from build123d import *

# Parameters (mm, degrees)
SKETCH1_R           = 4
SKETCH1_R_2         = 1.85
BOSS_EXTRUDE1_DEPTH = 2.3368


with BuildPart() as part:
    # Sketch1 → Boss-Extrude1 (new body)
    with BuildSketch(Plane.XY):
        with BuildLine():
            Line((-29.579916475, -5.002853321), (-33.915090683, 20.629337502))
            ThreePointArc((-33.915090683, 20.629337502), (-33.978735385, 21.133158673), (-34, 21.640538448))
            Line((-34, 21.640538448), (-34, 55.247304326))
            ThreePointArc((-34, 55.247304326), (-33.538424872, 57.567799195), (-32.223970118, 59.535019756))
            Line((-32.223970118, 59.535019756), (-9.899494937, 81.859494937))
            ThreePointArc((-9.899494937, 81.859494937), (0, 85.96), (9.899494937, 81.859494937))
            Line((9.899494937, 81.859494937), (32.223970118, 59.535019756))
            ThreePointArc((32.223970118, 59.535019756), (33.538424872, 57.567799195), (34, 55.247304326))
            Line((34, 55.247304326), (34, 21.640538448))
            ThreePointArc((34, 21.640538448), (33.978735385, 21.133158673), (33.915090683, 20.629337502))
            Line((33.915090683, 20.629337502), (29.579916475, -5.002853321))
            ThreePointArc((29.579916475, -5.002853321), (0, -30), (-29.579916475, -5.002853321))
        make_face()
        Circle(SKETCH1_R, mode=Mode.SUBTRACT)
        with Locations((0, 8)):
            Circle(SKETCH1_R_2, mode=Mode.SUBTRACT)
        with Locations((-8, 0)):
            Circle(SKETCH1_R_2, mode=Mode.SUBTRACT)
        with Locations((0, -8)):
            Circle(SKETCH1_R_2, mode=Mode.SUBTRACT)
        with Locations((8, 0)):
            Circle(SKETCH1_R_2, mode=Mode.SUBTRACT)
        with Locations((0, 71.96)):
            Circle(SKETCH1_R, mode=Mode.SUBTRACT)
        with Locations((-29.2625, 32)):
            Circle(SKETCH1_R_2, mode=Mode.SUBTRACT)
        with Locations((29.2625, 43.5)):
            Circle(SKETCH1_R_2, mode=Mode.SUBTRACT)
        with Locations((29.2625, 32)):
            Circle(SKETCH1_R_2, mode=Mode.SUBTRACT)
        with Locations((-29.2625, 43.5)):
            Circle(SKETCH1_R_2, mode=Mode.SUBTRACT)
    extrude(amount=BOSS_EXTRUDE1_DEPTH)


solid = part.part
Geometry: final body of the model. Coordinates: model frame, mm. Coordinates: 2 decimals unless noted, no trailing zeros. Loops run counter-clockwise (first coordinate to the right, second up) from the corner with the lowest first, then second, coordinate; pieces in that order, holes last. Notation, with made-up numbers: M -8,50 L 44,50 A29 cw 44,73 Z; hole C -17.75,65.25 d8. An arc over 180 degrees is marked long. One line per item, written item: value. Start each with the question number.
1) Pin query (flat end, axial travel): P1, Ø2, axis at x = 0, y = 8, coming from the -Z side; P2, Ø4.5, axis at x = 29.26, y = 43.5, coming from the +Z side. Return the tip coordinate at first contact, or that it passes through.
2) Material intervals for L1, parallel to Y at x = 0, z = 1.55; L2, parallel to Y at x = 1.5, z = 0.4; L3, parallel to X at y = 42, z = 1.3, sorted ascending. Write a range as from..to.
3) Cut plane A-A (x = 0). Return loops of the section in (y, z).
4) Cut plane B-B (y = 32). Return loops of the section in (x, z).
5) Draft query along Y for faces 1 (the cylindrical face through (-33.55, 57.54, 1.15)), 2 (the cylindrical face through (-0.401, 6.194, 1.152)), 3 (the flat face through (-31.717, 7.634, 1.152)). Return one class per face: released by +Y, released by -Y, zero draft, split by the parting line, or undercut.
6) Cut plane C-C (z = 1.1). Count the separate pieces of the cut face and the enclosed holes in it, then the cut area to 3 significant figures.
7) Cut plane D-D (y = -8). Return loops of the section in (x, z).
Evaluation:
1. P1: through
1. P2: z = 2.34
2. L1: -30..-9.85, -6.15..-4, 4..6.15, 9.85..67.96, 75.96..85.96
2. L2: -29.96..-9.08, -6.92..-3.71, 3.71..6.92, 9.08..68.25, 75.67..85.88
2. L3: -34..-30.35, -28.18..28.18, 30.35..34
3. outline: M -30,0 L -9.85,0 L -9.85,2.34 L -30,2.34 Z; M -6.15,0 L -4,0 L -4,2.34 L -6.15,2.34 Z; M 4,0 L 6.15,0 L 6.15,2.34 L 4,2.34 Z; M 9.85,0 L 67.96,0 L 67.96,2.34 L 9.85,2.34 Z; M 75.96,0 L 85.96,0 L 85.96,2.34 L 75.96,2.34 Z
4. outline: M -34,0 L -31.11,0 L -31.11,2.34 L -34,2.34 Z; M -27.41,0 L 27.41,0 L 27.41,2.34 L -27.41,2.34 Z; M 31.11,0 L 34,0 L 34,2.34 L 31.11,2.34 Z
5. face 1: released by +Y
5. face 2: undercut
5. face 3: released by -Y
6. separate pieces: 1
6. enclosed holes: 10
6. area: 6,190 mm^2
7. outline: M -28.91,0 L -1.85,0 L -1.85,2.34 L -28.91,2.34 Z; M 1.85,0 L 28.91,0 L 28.91,2.34 L 1.85,2.34 Z
